Design review of the part shown in the three views and the two pictorial views. Dimensions are in mm from the part's minimum x, y and z. A direction names the side the tool comes from. Round coordinates to 2 decimals unless told otherwise and drop trailing zeros. Loops run counter-clockwise (first coordinate to the right, second up) from the corner with the lowest first, then second, coordinate; pieces in that order, holes last. Notation, with made-up numbers: (82.25, 3.25) -> (127.25, 3.25) arc R5 cw to (127.25, 8.25) -> close; hole circle Ø10 at (6, -33.5). An arc over 180 degrees is marked (long way). Return JSON: item names as keys, results as strings. Group by question number.
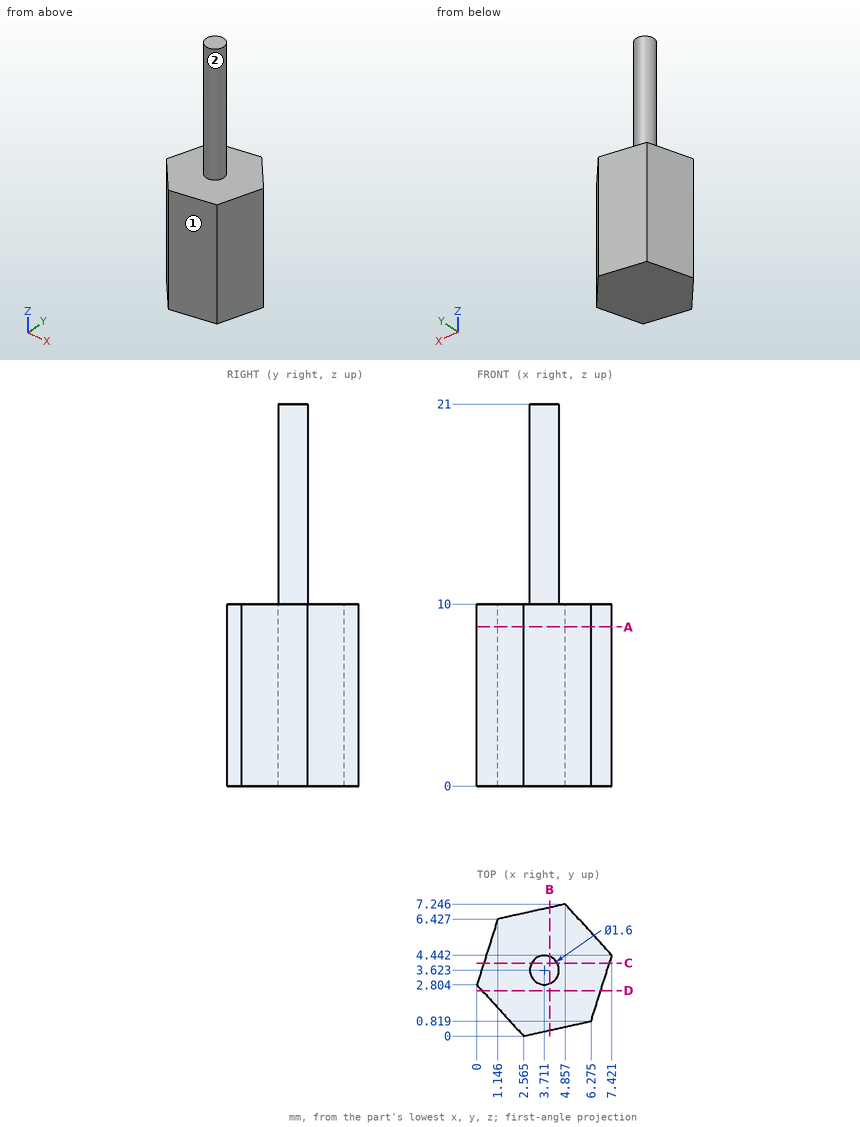
1. We need section D-D, the plane y = 2.5. Write out the cut boundary in (x, z), then the cut area to 3 significant figures.
2. We need section B-B, the plane x = 4. Write out the cut boundary in (y, z).
3. Wall thickness on line 1 (Z direction, x = 4.25, y = 6.25); line 2 (X direction, y = 4, z = 12.5) (1 decimal); line 3 (Y direction, x = 4.5, z = 3.75): over which ranges is each line inside the solid? List them lowest first.
4. We need section A-A, the plane z = 8.75. Write out the cut boundary in (x, y) (1 decimal).
5. We need section C-C, the plane y = 4. Write out the cut boundary in (x, z) (1 decimal).
6. Tool access review of the marked faces 1 and 2: name each direction out of +Z, -Z, +X, -X, +Y, -Y from which nothing blocks a thin tool from reaching the whole face with its end or side.
7. For P1, Ø4, axis at x = 2.5, z = 19, coming from the +Y side; P2, Ø1.5, axis at x = 6.5, y = 6, coming from the +Z side, all flat-tipped, find the tip position at first contact; note any pin that passes through.
Check sheet entries:
{
 "1": {"outline": "(0.28, 0) -> (6.81, 0) -> (6.81, 10) -> (0.28, 10) -> close", "area": "65.3 mm²"},
 "2": {"outline": "(0.32, 0) -> (7.06, 0) -> (7.06, 10) -> (4.37, 10) -> (4.37, 21) -> (2.88, 21) -> (2.88, 10) -> (0.32, 10) -> close"},
 "3": {"line 1": "z = 0 to 10", "line 2": "x = 3 to 4.4", "line 3": "y = 0.43 to 7.17"},
 "4": {"outline": "(0, 2.8) -> (2.6, 0) -> (6.3, 0.8) -> (7.4, 4.4) -> (4.9, 7.2) -> (1.1, 6.4) -> close"},
 "5": {"outline": "(0.4, 0) -> (7.3, 0) -> (7.3, 10) -> (4.4, 10) -> (4.4, 21) -> (3, 21) -> (3, 10) -> (0.4, 10) -> close"},
 "6": {"face 1": "+Z, -Z, +X, -Y", "face 2": "+Z"},
 "7": {"P1": "stops at y = 4.42", "P2": "stops at z = 10"}
}
